```python
from build123d import *

# Parameters (mm, degrees)
SKETCH_R     = 42
PAD_DEPTH    = 7
SKETCH003_R  = 27
PAD001_DEPTH = 3.4
SKETCH004_R  = 3
HOLE_DEPTH   = 25


with BuildPart() as part:
    # Sketch → Pad (new body)
    with BuildSketch(Plane.XY):
        Circle(SKETCH_R)
        with BuildLine():
            Line((-2.9, 14.84438), (-2.9, 12.84438))
            Line((-2.9, 12.84438), (2.9, 12.84438))
            Line((2.9, 12.84438), (2.9, 14.84438))
            ThreePointArc((-2.9, 14.84438), (0, -15.125), (2.9, 14.84438))
        make_face(mode=Mode.SUBTRACT)
    extrude(amount=PAD_DEPTH)

    # Sketch003 (on Face7 of Pad) → Pad001 (join)
    with BuildSketch(Plane.XY.offset(7)):
        Circle(SKETCH003_R)
        with BuildLine():
            ThreePointArc((-2.9, 14.84438), (0, -15.125), (2.9, 14.84438))
            Line((2.9, 12.84438), (2.9, 14.84438))
            Line((-2.9, 12.84438), (2.9, 12.84438))
            Line((-2.9, 14.84438), (-2.9, 12.84438))
        make_face(mode=Mode.SUBTRACT)
    extrude(amount=PAD001_DEPTH)

    # Sketch004 (on Face3 of Pad001) → Hole (cut)
    with BuildSketch(Plane.XY.offset(7)):
        with Locations((0, 32.5)):
            Circle(SKETCH004_R)
        with Locations((0, -32.5)):
            Circle(SKETCH004_R)
        with Locations((32.5, 0)):
            Circle(SKETCH004_R)
        with Locations((-32.5, 0)):
            Circle(SKETCH004_R)
    extrude(amount=-HOLE_DEPTH, mode=Mode.SUBTRACT)


solid = part.part
```
Build history of the part. All positions in model axes, mm. A direction names the side the tool comes from. Round coordinates to 2 decimals unless told otherwise and drop trailing zeros. Loops run counter-clockwise (first coordinate to the right, second up) from the corner with the lowest first, then second, coordinate; pieces in that order, holes last.
Item 1: Drill centre lines: line 1 along Y through (x, z) = (0, 2.5) (3 decimals); line 2 along Z through (x, y) = (11.5, -37.5); line 3 along Y through (x, z) = (-9, 8.5). Where is each one in solid material? Low to high.
Item 2: Saw through at A-A (y = 0). List the corners of the cut face in (x, z) (3 decimals).
Item 3: Saw through at D-D (y = 8.5). List the corners of the cut face in (x, z), then the cut area to 3 significant figures.
Item 4: Two-plate mould, pull along X, no slides. Class faces 1 (the face through (-0.6, -27.4, 7)), 2 (the face through (29.5, 0.1, 3.5)), 3 (the face through (40.06, 12.62, 3.45)): released by +X, released by -X, zero draft, split by the parting line, or undercut.
Item 5: Pin check, flat tips, straight feed: P1, Ø2, axis at y = 14.5, z = 6.5, coming from the +X side; P2, Ø2, axis at x = 10, z = 2.5, coming from the +Y side; P3, Ø6, axis at y = 15.5, z = 7.5, coming from the +X side. Stop position of each tip, or through.
Item 6: Saw through at C-C (z = 5.5). List the corners of the cut face in (x, y) (3 decimals), then the cut area to 3 significant figures.
Item 7: Saw through at B-B (x = 0). List the corners of the cut face in (y, z) (3 decimals).
Item 8: Which spindle directions (+Z, -Z, +X, -X, +Y, -Y) get a long thin tool onto all of the face, cutting with end or side? Do faces 4 (the face through (18, 1, 0)), 5 (the face through (-5.85, -26.36, 8.68)), 6 (the face through (2.9, 14, 5)). Say none if no direction does.
Worked answers:
1. line 1: y = -42 to -35.5, -29.5 to -15.125, 12.844 to 29.5, 35.5 to 42
1. line 2: z = 0 to 7
1. line 3: y = -25.46 to -12.16, 12.16 to 25.46
2. outline: (-42, 0) - (-35.5, 0) - (-35.5, 7) - (-42, 7) - close; (-29.5, 0) - (-15.125, 0) - (-15.125, 10.4) - (-27, 10.4) - (-27, 7) - (-29.5, 7) - close; (15.125, 0) - (29.5, 0) - (29.5, 7) - (27, 7) - (27, 10.4) - (15.125, 10.4) - close; (35.5, 0) - (42, 0) - (42, 7) - (35.5, 7) - close
3. outline: (-41.13, 0) - (-12.51, 0) - (-12.51, 10.4) - (-25.63, 10.4) - (-25.63, 7) - (-41.13, 7) - close; (12.51, 0) - (41.13, 0) - (41.13, 7) - (25.63, 7) - (25.63, 10.4) - (12.51, 10.4) - close
3. area: 490 mm2
4. face 1: zero draft
4. face 2: undercut
4. face 3: split by the parting line
5. P1: stops at x = 39.77
5. P2: stops at y = 41.02
5. P3: stops at x = 40.08
6. outline: circle Ø84 at (0, 0); hole circle Ø6 at (-32.5, 0); hole circle Ø6 at (0, -32.5); hole circle Ø6 at (0, 32.5); hole (-2.9, 12.844) - (-2.9, 14.844) arc R15.125 ccw (long way) to (2.9, 14.844) - (2.9, 12.844) - close; hole circle Ø6 at (32.5, 0)
6. area: 4,720 mm2
7. outline: (-42, 0) - (-35.5, 0) - (-35.5, 7) - (-42, 7) - close; (-29.5, 0) - (-15.125, 0) - (-15.125, 10.4) - (-27, 10.4) - (-27, 7) - (-29.5, 7) - close; (12.844, 0) - (29.5, 0) - (29.5, 7) - (27, 7) - (27, 10.4) - (12.844, 10.4) - close; (35.5, 0) - (42, 0) - (42, 7) - (35.5, 7) - close
8. face 4: -Z, +X, -X, +Y, -Y
8. face 5: +Z
8. face 6: +Z, -Z
